The drawing under review shows one solid part. Ordinate dimensions are in mm from its lowest x, y, z. A direction names the side the tool comes from. Coordinates: 2 decimals unless noted, no trailing zeros. Order: outer loops, then holes, each group sorted by start corner. A loop starts at its lowest first (then second) coordinate and runs counter-clockwise, first axis right, second up. Notation, with made-up numbers: (28.25, 58) -> (45.25, 58) arc R27 cw to (45.25, 75) -> close; hole circle Ø6 at (30.5, 2.25). An arc over 180 degrees is marked (long way). Use one line per item in the form item = value.
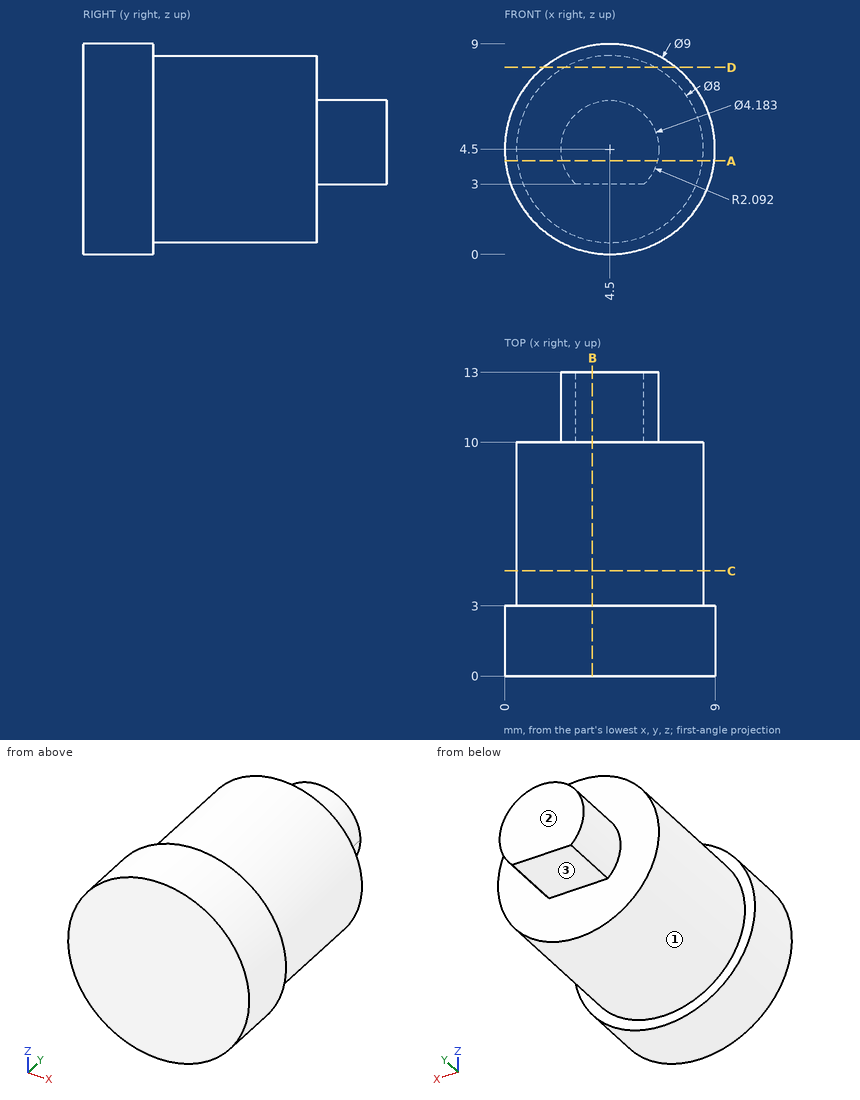
Item 1: Clearance check with flat-ended pins moving along their axes: pin 1 (0.9 mm diameter, centred on x = 4, y = 11.5, fed in from -Z); pin 2 (1 mm diameter, centred on y = 5, z = 1, fed in from +X) (1 decimal); pin 3 (4 mm diameter, centred on y = 8, z = 6.5, fed in from -X). State where each tip first meets the part, or that it passes through.
Results found:
pin_1 = 3
pin_2 = 7.1
pin_3 = 0.5
Item 2: Tool access review of the marked faces 1, 2 and 3: name each direction out of +Z, -Z, +X, -X, +Y, -Y from which nothing blocks a thin tool from reaching the whole face with its end or side.
Results found:
face_1 = +Y
face_2 = +Z, -Z, +X, -X, +Y
face_3 = -Z, +X, -X, +Y
Item 3: We need section D-D (z = 8). Write out the cut boundary in (x, y), plus the area to 3 significant figures.
Results found:
outline = (1.67, 0) -> (7.33, 0) -> (7.33, 3) -> (6.44, 3) -> (6.44, 10) -> (2.56, 10) -> (2.56, 3) -> (1.67, 3) -> close
area = 44.1 mm²
Item 4: We need section C-C (y = 4.5). Write out the cut boundary in (x, z).
Results found:
outline = circle Ø8 at (4.5, 4.5)
Item 5: To check wall thickness, follow L1, parallel to Y at x = 4, z = 7.5; L2, parallel to X at y = 11, z = 4.5; L3, parallel to Z at x = 4.5, y = 8.75. State the ranges of each line that lie inside material, in increasing order. Write a range as from..to.
Results found:
L1 = 0..10
L2 = 2.41..6.59
L3 = 0.5..8.5
Item 6: We need section B-B (x = 3.75). Write out the cut boundary in (y, z).
Results found:
outline = (0, 0.06) -> (3, 0.06) -> (3, 0.57) -> (10, 0.57) -> (10, 3) -> (13, 3) -> (13, 6.45) -> (10, 6.45) -> (10, 8.43) -> (3, 8.43) -> (3, 8.94) -> (0, 8.94) -> close
Item 7: We need section A-A (z = 4). Write out the cut boundary in (x, y).
Results found:
outline = (0.03, 0) -> (8.97, 0) -> (8.97, 3) -> (8.47, 3) -> (8.47, 10) -> (6.53, 10) -> (6.53, 13) -> (2.47, 13) -> (2.47, 10) -> (0.53, 10) -> (0.53, 3) -> (0.03, 3) -> close
